from build123d import *

# Parameters (mm, degrees)
F0_R        = 10.31875
F0_R_2      = 2.15265
F1_DEPTH    = 3.175
F2_W        = 11.2655872395
F2_H        = 11.2655872395
F2_R        = 2.15265
F3_DEPTH    = 7.9375
F4_R        = 1.35255
F5_REACH    = 19.7781327273
F6_T1_DEPTH = 22.01948225
F7_W        = 0.79375
F7_H        = 1.5875


# Not quite as in the source:
# - a fillet or chamfer that OpenCascade refuses, or shapes differently, is made with other operations: its cross-section is extruded or revolved along the edge and cut away or added


with BuildPart() as f1:
    # F0 (on Top) → F1 (new body)
    with BuildSketch(Plane.XY):
        Circle(F0_R)
        Circle(F0_R_2, mode=Mode.SUBTRACT)
    extrude(amount=F1_DEPTH)

    # F2 (on face) → F3 (join)
    with BuildSketch(Plane.XY.offset(3.175)):
        Rectangle(F2_W, F2_H)
        Circle(F2_R, mode=Mode.SUBTRACT)
    extrude(amount=F3_DEPTH)

    f5_end = f1.faces().sort_by_distance((-2.15265, 0, 5.55625))[0]
    # F4 (on face) → F5 (cut, up to a face of the model that its end follows)
    with BuildSketch(Plane.XZ.offset(5.6327936197)):
        with Locations((0, 7.14375)):
            Circle(F4_R)
    f5_long = extrude(amount=-F5_REACH, mode=Mode.PRIVATE)
    add(split(f5_long, bisect_by=f5_end, keep=Keep.ALL, mode=Mode.PRIVATE).solids().sort_by_distance((0, -5.6327936197, 7.14375))[0], mode=Mode.SUBTRACT)

    # F6: fillet of radius 5.6327929 on 4 edges, made by hand

    # F6_s2 → F6_t1 (cut)
    with BuildSketch(Plane.XY.offset(3.175)):
        with BuildLine():
            ThreePointArc((-5.6327936197, -7.197e-07), (-3.9829867763, -3.9829867763), (-7.197e-07, -5.6327936197))
            Line((-7.197e-07, -5.6327936197), (-5.6327936197, -5.6327936197))
            Line((-5.6327936197, -5.6327936197), (-5.6327936197, -7.197e-07))
        make_face()
        with BuildLine():
            ThreePointArc((7.197e-07, -5.6327936197), (3.9829867763, -3.9829867763), (5.6327936197, -7.197e-07))
            Line((5.6327936197, -7.197e-07), (5.6327936197, -5.6327936197))
            Line((5.6327936197, -5.6327936197), (7.197e-07, -5.6327936197))
        make_face()
        with BuildLine():
            ThreePointArc((7.197e-07, 5.6327936197), (3.9829867763, 3.9829867763), (5.6327936197, 7.197e-07))
            Line((5.6327936197, 7.197e-07), (5.6327936197, 5.6327936197))
            Line((5.6327936197, 5.6327936197), (7.197e-07, 5.6327936197))
        make_face()
        with BuildLine():
            ThreePointArc((-7.197e-07, 5.6327936197), (-3.9829867763, 3.9829867763), (-5.6327936197, 7.197e-07))
            Line((-5.6327936197, 7.197e-07), (-5.6327936197, 5.6327936197))
            Line((-5.6327936197, 5.6327936197), (-7.197e-07, 5.6327936197))
        make_face()
    extrude(amount=F6_T1_DEPTH, mode=Mode.SUBTRACT)

    # F7 (on Front) → F8 (revolve, cut)
    with BuildSketch(Plane.XZ):
        with Locations((9.921875, 1.5875)):
            Rectangle(F7_W, F7_H)
    revolve(axis=Axis((0, 0, 0), (0, 0, 1)), mode=Mode.SUBTRACT)


solid = f1.part
Could you check a few things on this model? Use its own coordinates, in mm. A direction names the side the tool comes from. Give positions to 0.01 mm unless a question says otherwise; leave off trailing zeros. Order: outer loops, then holes, each group sorted by start corner. A loop starts at its lowest first (then second) coordinate and runs counter-clockwise, first axis right, second up.
Item 1: If we section it at B-B, the plane y = -4.25: Write out the boundary of the cut face in (x, z) (1 decimal), plus the area to 3 significant figures.
Item 2: If we section it at C-C, the plane y = -7.5: Write out the boundary of the cut face in (x, z) (3 decimals).
Item 3: For faces 1 (the face through (-7, -7, 0.794)), 2 (the face through (3.939, 4.027, 7.088)), 3 (the face through (-3.939, 4.027, 7.088)), 4 (the face through (-4.027, -3.939, 7.088)), which set-ups out of +Z, -Z, +X, -X, +Y, -Y let a thin tool reach every point of the face, with its end or its side?
Item 4: I need wall thicknesses on line 1 (Z direction, x = 9.25, y = 4) (3 decimals); line 2 (Z direction, x = 0, y = -2.9); line 3 (Z direction, x = 3.75, y = 7.75) (3 decimals). Which ranges of each line are inside material? Lowest first, please.
Item 5: I'm going to push flat-ended pins straight in: pin 1 (1 mm diameter, centred on x = -2, z = 6.5, fed in from +Y); pin 2 (1 mm diameter, centred on x = -4.5, z = 7, fed in from -Y); pin 3 (1.5 mm diameter, centred on y = -6, z = 3, fed in from +X). Where does each tip first touch, or does it pass through?
Item 6: If we section it at D-D, the plane x = 3: Write out the boundary of the cut face in (y, z) (1 decimal).
Item 7: If we mould it in two halves opening along Z, with no side actions, what happens to faces 5 (the face through (-0.1, -2.4, 11.112)), 6 (the face through (-1.35, -3.68, 7.2)), 7 (the face through (-2.237, -10.073, 2.773))? For each: pulls with the +Z half, pulls with the -Z half, needs draft (parallel to the pull), parting line crosses it, or undercut.
Values:
1. outline: (-9.4, 0) - (9.4, 0) - (9.4, 0.8) - (8.5, 0.8) - (8.5, 2.4) - (9.4, 2.4) - (9.4, 3.2) - (3.7, 3.2) - (3.7, 11.1) - (-3.7, 11.1) - (-3.7, 3.2) - (-9.4, 3.2) - (-9.4, 2.4) - (-8.5, 2.4) - (-8.5, 0.8) - (-9.4, 0.8) - close; hole circle Ø2.7 at (0, 7.1)
1. area: 110 mm2
2. outline: (-7.087, 0) - (7.087, 0) - (7.087, 0.794) - (5.872, 0.794) - (5.872, 2.381) - (7.087, 2.381) - (7.087, 3.175) - (-7.087, 3.175) - (-7.087, 2.381) - (-5.872, 2.381) - (-5.872, 0.794) - (-7.087, 0.794) - close
3. face 1: none
3. face 2: +Z, +X, +Y
3. face 3: +Z, -X, +Y
3. face 4: +Z, -X, -Y
4. line 1: z = 0 to 0.794, 2.381 to 3.175
4. line 2: z = 0 to 5.79, 8.5 to 11.11
4. line 3: z = 0 to 3.175
5. pin 1: stops at y = 5.43
5. pin 2: stops at y = -3.97
5. pin 3: stops at x = 8.88
6. outline: (-9.9, 0) - (9.9, 0) - (9.9, 0.8) - (9, 0.8) - (9, 2.4) - (9.9, 2.4) - (9.9, 3.2) - (4.8, 3.2) - (4.8, 11.1) - (-4.8, 11.1) - (-4.8, 3.2) - (-9.9, 3.2) - (-9.9, 2.4) - (-9, 2.4) - (-9, 0.8) - (-9.9, 0.8) - close
7. face 5: pulls with the +Z half
7. face 6: undercut
7. face 7: needs draft
